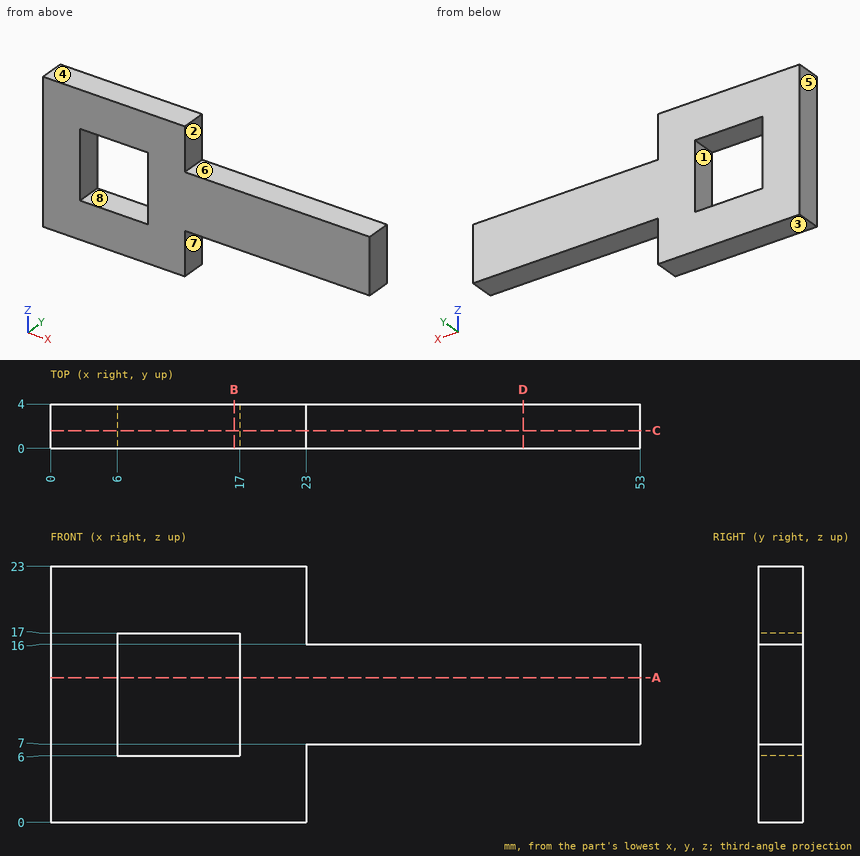
The figure shows three views and two pictorial views of one solid part (mm, origin at its lowest corner). Answer the questions. A direction names the side the tool comes from. Round coordinates to 2 decimals unless told otherwise and drop trailing zeros. Order: outer loops, then holes, each group sorted by start corner. A loop starts at its lowest first (then second) coordinate and runs counter-clockwise, first axis right, second up. Notation, with made-up numbers: (87, 11) -> (113, 11) arc R25 ccw to (113, 49) -> close; hole circle Ø2 at (-12.75, -35.5). An arc over 180 degrees is marked (long way). One line per item, written item: value.
Item 1: Find section A-A, the plane z = 13. Give the vertices of the cut face in (x, y), then the cut area to 3 significant figures.
Taken from the geometry:
outline: (0, 0) -> (6, 0) -> (6, 4) -> (0, 4) -> close; (17, 0) -> (53, 0) -> (53, 4) -> (17, 4) -> close
area: 168 mm2
Item 2: Given P1, Ø1.5, axis at y = 1, z = 18.5, coming from the +X side; P2, Ø1, axis at x = 26, y = 2.5, coming from the +Z side, each flat-ended and moving along its own axis, determine where each tip first touches the part or whether it passes through.
Taken from the geometry:
P1: stops at x = 23
P2: stops at z = 16
Item 3: Find section C-C, the plane y = 1.6. Give the vertices of the cut face in (x, z).
Taken from the geometry:
outline: (0, 0) -> (23, 0) -> (23, 7) -> (53, 7) -> (53, 16) -> (23, 16) -> (23, 23) -> (0, 23) -> close; hole (6, 6) -> (17, 6) -> (17, 17) -> (6, 17) -> close
Item 4: For the marked faces 5, 6, 7 and 8, determine the directions among +Z, -Z, +X, -X, +Y, -Y from which every point of the face is accessible in a straight line to the end or side of a thin tool.
Taken from the geometry:
face 5: +Z, -Z, -X, +Y, -Y
face 6: +Z, +X, +Y, -Y
face 7: -Z, +X, +Y, -Y
face 8: +Y, -Y
Item 5: Straight lines are drawn through the part: L1, parallel to X at y = 1.9, z = 11.75; L2, parallel to X at y = 2.3, z = 6.75. For each, find the intervals that lie inside material, in ascending order.
Taken from the geometry:
L1: x = 0 to 6, 17 to 53
L2: x = 0 to 6, 17 to 23
Item 6: Find section D-D, the plane x = 42.5. Give the vertices of the cut face in (y, z).
Taken from the geometry:
outline: (0, 7) -> (4, 7) -> (4, 16) -> (0, 16) -> close
Item 7: For a pull along Z with two mould halves and no side action, classify the marked faces 1, 2, 3 and 4 as released by +Z, released by -Z, zero draft, split by the parting line, or undercut.
Taken from the geometry:
face 1: undercut
face 2: zero draft
face 3: released by -Z
face 4: released by +Z
Item 8: Find section B-B, the plane x = 16.5. Give the vertices of the cut face in (y, z).
Taken from the geometry:
outline: (0, 0) -> (4, 0) -> (4, 6) -> (0, 6) -> close; (0, 17) -> (4, 17) -> (4, 23) -> (0, 23) -> close
